from build123d import *

# Parameters (mm, degrees)
SKETCH1_W           = 119.48
SKETCH1_H           = 177.8
BOSS_EXTRUDE1_DEPTH = 5.13
CUT_EXTRUDE1_DEPTH  = 5.13
SKETCH3_W           = 88
SKETCH3_H           = 8
VENTS_DEPTH         = 5.13
VENTS_PATTERN_COUNT = 5
VENTS_PATTERN_PITCH = 16
SKETCH4_W           = 5.13
SKETCH4_H           = 58.88
BOSS_EXTRUDE2_DEPTH = 5.13
SKETCH5_W           = 5.13
SKETCH5_H           = 58.88
BOSS_EXTRUDE3_DEPTH = 5.13


with BuildPart() as part:
    # Sketch1 → Boss-Extrude1 (new body)
    with BuildSketch(Plane(origin=(0, 0, 0), x_dir=(0, 0, -1), z_dir=(1, 0, 0))):
        with Locations((24.047197546, -50.943101868)):
            Rectangle(SKETCH1_W, SKETCH1_H)
    extrude(amount=BOSS_EXTRUDE1_DEPTH)

    # Sketch2 → Cut-Extrude1 (cut)
    with BuildSketch(Plane(origin=(5.13, 0, 0), x_dir=(0, 0, -1), z_dir=(1, 0, 0))):
        Polygon((-26.892802454, 37.956898132), (-23.895802454, 37.956898132), (-23.895802454, 33.961898132), (-22.536802454, 33.961898132), (-22.536802454, 31.794898132), (-23.895802454, 31.794898132), (-23.895802454, 25.587898132), (-26.892802454, 25.587898132), (-26.892802454, 31.794898132), (-28.251802454, 31.794898132), (-28.251802454, 33.961898132), (-26.892802454, 33.961898132), align=None)
        Polygon((71.987197546, 33.961898132), (71.987197546, 37.956898132), (74.984197546, 37.956898132), (74.984197546, 33.961898132), (76.343197546, 33.961898132), (76.343197546, 31.794898132), (74.984197546, 31.794898132), (74.984197546, 25.587898132), (71.987197546, 25.587898132), (71.987197546, 31.794898132), (70.628197546, 31.794898132), (70.628197546, 33.961898132), align=None)
        Polygon((76.343197546, -133.681101868), (74.984197546, -133.681101868), (74.984197546, -127.474101868), (71.987197546, -127.474101868), (71.987197546, -133.681101868), (70.628197546, -133.681101868), (70.628197546, -135.848101868), (71.987197546, -135.848101868), (71.987197546, -139.843101868), (74.984197546, -139.843101868), (74.984197546, -135.848101868), (76.343197546, -135.848101868), align=None)
        Polygon((-26.892802454, -139.843101868), (-23.895802454, -139.843101868), (-23.895802454, -135.848101868), (-22.536802454, -135.848101868), (-22.536802454, -133.681101868), (-23.895802454, -133.681101868), (-23.895802454, -127.474101868), (-26.892802454, -127.474101868), (-26.892802454, -133.681101868), (-28.251802454, -133.681101868), (-28.251802454, -135.848101868), (-26.892802454, -135.848101868), align=None)
    extrude(amount=-CUT_EXTRUDE1_DEPTH, mode=Mode.SUBTRACT)

    # Sketch3 → Vents (cut)
    with BuildSketch(Plane.ZY):
        with Locations((-24.047197546, -16.043101868)):
            Rectangle(SKETCH3_W, SKETCH3_H)
    vents = extrude(amount=-VENTS_DEPTH, mode=Mode.SUBTRACT)

    # Vents pattern: Vents ×5
    with Locations(*[(0, -i * VENTS_PATTERN_PITCH, 0) for i in range(1, VENTS_PATTERN_COUNT)]):
        add(vents, mode=Mode.SUBTRACT)

    # Sketch4 → Boss-Extrude2 (add)
    with BuildSketch(Plane(origin=(0, 37.956898132, 0), x_dir=(1, 0, 0), z_dir=(0, 1, 0))):
        with Locations((2.565, 24.047197546)):
            Rectangle(SKETCH4_W, SKETCH4_H)
    extrude(amount=BOSS_EXTRUDE2_DEPTH)

    # Sketch5 → Boss-Extrude3 (add)
    with BuildSketch(Plane.XZ.offset(139.843101868)):
        with Locations((2.565, -24.047197546)):
            Rectangle(SKETCH5_W, SKETCH5_H)
    extrude(amount=BOSS_EXTRUDE3_DEPTH)


solid = part.part
CAD build for the part. Positions are in the model's coordinates, mm. A direction names the side the tool comes from. Give positions to 0.01 mm unless a question says otherwise; leave off trailing zeros. Order: outer loops, then holes, each group sorted by start corner. A loop starts at its lowest first (then second) coordinate and runs counter-clockwise, first axis right, second up. Notation, with made-up numbers: (-24.5, 57) - (16.5, 57) arc R31 cw to (16.5, 96) - close; hole circle Ø5 at (76, 33). An arc over 180 degrees is marked (long way). Answer in a Markdown table with one row per item.
1. Saw through at D-D, the plane x = 3.1. Count the separate pieces of the cut face and the enclosed holes in it, plus the area to 3 significant figures.
Data:
| item | result |
|---|---|
| separate pieces | 1 |
| enclosed holes | 5 |
| area | 18,200 mm² |
2. Saw through at A-A, the plane z = -10. Give the cut face in (x, y).
Data:
| item | result |
|---|---|
| outline | (0, -144.97) - (5.13, -144.97) - (5.13, -84.04) - (0, -84.04) - close; (0, -76.04) - (5.13, -76.04) - (5.13, -68.04) - (0, -68.04) - close; (0, -60.04) - (5.13, -60.04) - (5.13, -52.04) - (0, -52.04) - close; (0, -44.04) - (5.13, -44.04) - (5.13, -36.04) - (0, -36.04) - close; (0, -28.04) - (5.13, -28.04) - (5.13, -20.04) - (0, -20.04) - close; (0, -12.04) - (5.13, -12.04) - (5.13, 43.09) - (0, 43.09) - close |
3. Flat gauge pins, fed straight in: pin 1 (0.7 mm diameter, centred on x = 1.5, z = -71, fed in from -Y); pin 2 (0.7 mm diameter, centred on x = 2.5, z = -76, fed in from +Y). Where does each tip first touch, or does it go through?
Data:
| item | result |
|---|---|
| pin 1 | stops at y = -139.84 |
| pin 2 | stops at y = 37.96 |
4. Saw through at C-C, the plane z = 12. Give the cut face in (x, y).
Data:
| item | result |
|---|---|
| outline | (0, -139.84) - (5.13, -139.84) - (5.13, -84.04) - (0, -84.04) - close; (0, -76.04) - (5.13, -76.04) - (5.13, -68.04) - (0, -68.04) - close; (0, -60.04) - (5.13, -60.04) - (5.13, -52.04) - (0, -52.04) - close; (0, -44.04) - (5.13, -44.04) - (5.13, -36.04) - (0, -36.04) - close; (0, -28.04) - (5.13, -28.04) - (5.13, -20.04) - (0, -20.04) - close; (0, -12.04) - (5.13, -12.04) - (5.13, 37.96) - (0, 37.96) - close |
5. Saw through at B-B, the plane y = 27.5. Give the cut face in (x, z).
Data:
| item | result |
|---|---|
| outline | (0, -83.79) - (5.13, -83.79) - (5.13, -74.98) - (0, -74.98) - close; (0, -71.99) - (5.13, -71.99) - (5.13, 23.9) - (0, 23.9) - close; (0, 26.89) - (5.13, 26.89) - (5.13, 35.69) - (0, 35.69) - close |
6. Pull direction Y, two halves, no side cores. Call faces 4 (the flat face through (3, -12.043, -25)), 5 (the flat face through (3, 37.957, 15)), 6 (the flat face through (3, 29, -74.984)), 7 (the flat face through (3, -20.043, -25)): pulls with the +Y half, pulls with the -Y half, needs draft (parallel to the pull), parting line crosses it, or undercut.
Data:
| item | result |
|---|---|
| face 4 | undercut |
| face 5 | pulls with the +Y half |
| face 6 | needs draft |
| face 7 | undercut |
7. Probe probe 1 along Z at (x, y) = (3.05, -129.5); probe 2 along Y at (x, z) = (4.7, -19); probe 3 along Y at (x, z) = (0.85, -62.5). List the from-to ranges inside material, lowest first. Write a range as [from, to].
Data:
| item | result |
|---|---|
| probe 1 | z = [-83.79, -74.98], [-71.99, 23.9], [26.89, 35.69] |
| probe 2 | y = [-144.97, -84.04], [-76.04, -68.04], [-60.04, -52.04], [-44.04, -36.04], [-28.04, -20.04], [-12.04, 43.09] |
| probe 3 | y = [-139.84, -84.04], [-76.04, -68.04], [-60.04, -52.04], [-44.04, -36.04], [-28.04, -20.04], [-12.04, 37.96] |
8. Tool access for faces 1 (the flat face through (3, -138, 23.896)), 2 (the flat face through (3, -84.043, -25)), 3 (the flat face through (3, -139.843, 15)): list every direction of +Z, -Z, +X, -X, +Y, -Y with a clear straight run to the whole face (end or side of a thin tool).
Data:
| item | result |
|---|---|
| face 1 | +X, -X, -Y |
| face 2 | +X, -X |
| face 3 | +Z, +X, -X, -Y |
